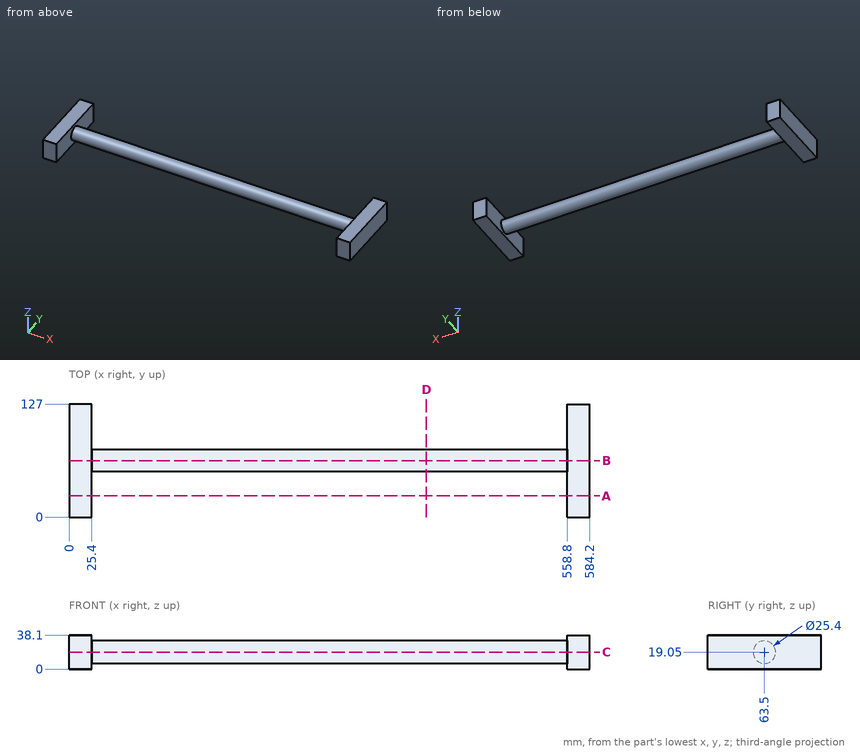
Design review of the part shown in the three views and the two pictorial views. Dimensions are in mm from the part's minimum x, y and z. Coordinates: 2 decimals unless noted, no trailing zeros. Order: outer loops, then holes, each group sorted by start corner. A loop starts at its lowest first (then second) coordinate and runs counter-clockwise, first axis right, second up.
Item 1: Take a section at B-B, the plane y = 63.5. Write out the cut boundary in (x, z), then the cut area to 3 significant figures.
Item 2: Take a section at C-C, the plane z = 19.05. Write out the cut boundary in (x, y), then the cut area to 3 significant figures.
Item 3: For pin 1 Ø12 at (x, z) = (510.5, 28) entering from -Y; pin 2 Ø10 at (x, z) = (498.5, 19) entering from -Y; pin 3 Ø1.5 at (x, z) = (305, 8) entering from +Y, all flat-tipped, find the tip position at first contact; note any pin that passes through.
Item 4: Take a section at A-A, the plane y = 24. Write out the cut boundary in (x, z), then the cut area to 3 significant figures.
Item 5: Take a section at D-D, the plane x = 401. Write out the cut boundary in (y, z).
Item 6: For line 1 (X direction, y = 50.5, z = 6); line 2 (Y direction, x = 335.5, z = 19); line 3 (Y direction, x = 474.5, z = 15), list the stretches that pass through material, from the lowest coordinate up.
The answers:
1. outline: (0, 0) - (25.4, 0) - (25.4, 6.35) - (558.8, 6.35) - (558.8, 0) - (584.2, 0) - (584.2, 38.1) - (558.8, 38.1) - (558.8, 31.75) - (25.4, 31.75) - (25.4, 38.1) - (0, 38.1) - close
1. area: 15,500 mm2
2. outline: (0, 0) - (25.4, 0) - (25.4, 50.8) - (558.8, 50.8) - (558.8, 0) - (584.2, 0) - (584.2, 127) - (558.8, 127) - (558.8, 76.2) - (25.4, 76.2) - (25.4, 127) - (0, 127) - close
2. area: 20,000 mm2
3. pin 1: stops at y = 51.15
3. pin 2: stops at y = 50.8
3. pin 3: stops at y = 70.93
4. outline: (0, 0) - (25.4, 0) - (25.4, 38.1) - (0, 38.1) - close; (558.8, 0) - (584.2, 0) - (584.2, 38.1) - (558.8, 38.1) - close
4. area: 1,940 mm2
5. outline: circle Ø25.4 at (63.5, 19.05)
6. line 1: x = 0 to 25.4, 558.8 to 584.2
6. line 2: y = 50.8 to 76.2
6. line 3: y = 51.46 to 75.54
